Can you work these out from the drawing? Everything is in mm from the part's minimum corner. Round coordinates to 2 decimals unless told otherwise and drop trailing zeros. Loops run counter-clockwise (first coordinate to the right, second up) from the corner with the lowest first, then second, coordinate; pieces in that order, holes last. Notation, with made-up numbers: M 2.5,83.5 L 30.5,83.5 A18 cw 30.5,94.5 Z; hole C -36,-0.5 d10. An arc over 180 degrees is marked long. Use a Markdown table: item, result.
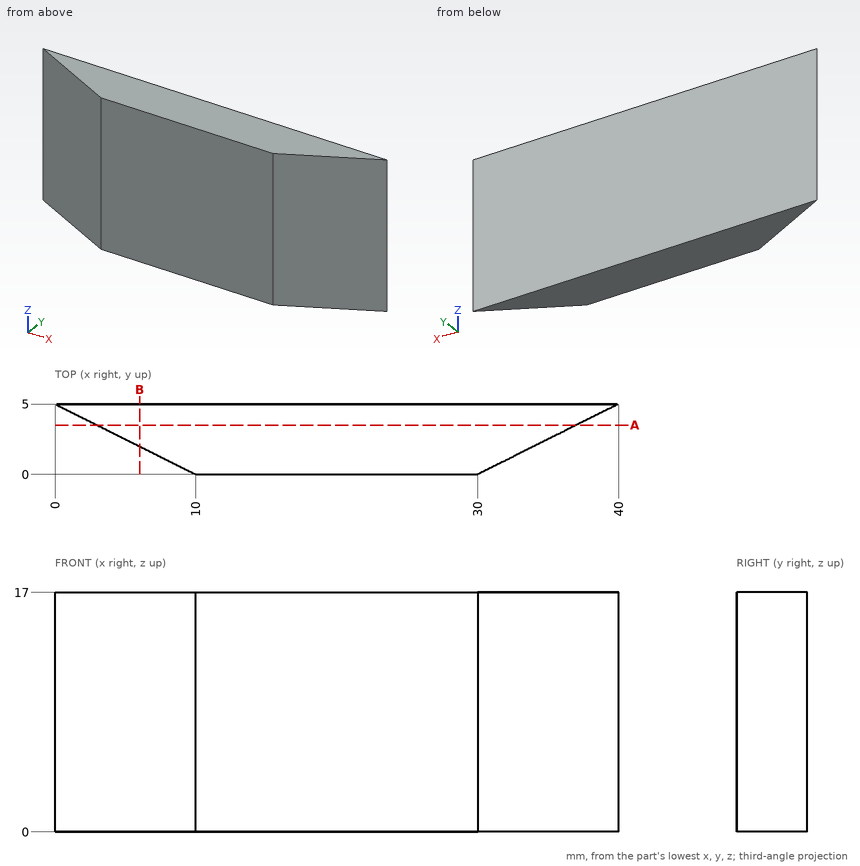
Q1. Will this pin go through, and if not, where does the flat tip stop? P1, Ø2, axis at y = 3, z = 3.5, coming from the +X side.
Return value:
| item | result |
|---|---|
| P1 | stops at x = 38 |
Q2. I need wall thicknesses on line 1 (X direction, y = 2.1, z = 14); line 2 (X direction, y = 1.7, z = 2.75); line 3 (Y direction, x = 6.5, z = 8.25). Which ranges of each line are inside material? Lowest first, please. Write a range as from..to.
Return value:
| item | result |
|---|---|
| line 1 | x = 5.8..34.2 |
| line 2 | x = 6.6..33.4 |
| line 3 | y = 1.75..5 |
Q3. Imagine slicing it at A-A, the plane y = 3.5. Please give me the cut outline in (x, z), then the cut area to 3 significant figures.
Return value:
| item | result |
|---|---|
| outline | M 3,0 L 37,0 L 37,17 L 3,17 Z |
| area | 578 mm^2 |
Q4. Imagine slicing it at B-B, the plane x = 6. Please give me the cut outline in (y, z).
Return value:
| item | result |
|---|---|
| outline | M 2,0 L 5,0 L 5,17 L 2,17 Z |
